Model file for the job. Use its own axes, mm. A direction names the side the tool comes from. Give positions to 0.01 mm unless a question says otherwise; leave off trailing zeros. Write each loop counter-clockwise with the first axis right and the second up, starting at its lowest first coordinate (ties: lowest second). Pieces come first, ordered by that corner, then holes.
```python
from build123d import *

# Parameters (mm, degrees)
SKETCH2_R           = 18.415
BOSS_EXTRUDE1_DEPTH = 70.104
SKETCH3_R           = 6.0325
BOSS_EXTRUDE2_DEPTH = 5.715
SKETCH5_R           = 3.01625
BOSS_EXTRUDE3_DEPTH = 14.986


with BuildPart() as part:
    # Sketch2 → Boss-Extrude1 (new body)
    with BuildSketch(Plane.XY):
        Circle(SKETCH2_R)
    extrude(amount=BOSS_EXTRUDE1_DEPTH)

    # Sketch3 → Boss-Extrude2 (add)
    with BuildSketch(Plane.XY.offset(70.104)):
        with Locations((0, -7.239)):
            Circle(SKETCH3_R)
    extrude(amount=BOSS_EXTRUDE2_DEPTH)

    # Sketch5 → Boss-Extrude3 (add)
    with BuildSketch(Plane.XY.offset(75.819)):
        with Locations((0, -7.239)):
            Circle(SKETCH5_R)
    extrude(amount=BOSS_EXTRUDE3_DEPTH)


solid = part.part
```
1. Slice it at A-A, the plane x = 0. Write the cut outline in (y, z) (1 decimal), and give its area (3 significant figures).
Calculated:
outline: (-18.4, 0) - (18.4, 0) - (18.4, 70.1) - (-1.2, 70.1) - (-1.2, 75.8) - (-4.2, 75.8) - (-4.2, 90.8) - (-10.3, 90.8) - (-10.3, 75.8) - (-13.3, 75.8) - (-13.3, 70.1) - (-18.4, 70.1) - close
area: 2,740 mm2
2. Probe probe 1 along Z at (x, y) = (12, 13.5); probe 2 along X at (y, z) = (-10.5, 53); probe 3 along X at (y, z) = (2, 14.5). List the from-to ranges inside material, lowest first.
Calculated:
probe 1: z = 0 to 70.1
probe 2: x = -15.13 to 15.13
probe 3: x = -18.31 to 18.31
3. Which spindle directions (+Z, -Z, +X, -X, +Y, -Y) get a long thin tool onto all of the face, cutting with end or side? Do faces 1 (the cylindrical face through (-14.61, -11.21, 34.56)), 2 (the flat face through (1, -4, 75.819)). Say none if no direction does.
Calculated:
face 1: +Z, -Z
face 2: +Z
4. Slice it at D-D, the plane y = -9. Write the cut outline in (x, z) (3 decimals).
Calculated:
outline: (-16.066, 0) - (16.066, 0) - (16.066, 70.104) - (5.77, 70.104) - (5.77, 75.819) - (2.449, 75.819) - (2.449, 90.805) - (-2.449, 90.805) - (-2.449, 75.819) - (-5.77, 75.819) - (-5.77, 70.104) - (-16.066, 70.104) - close
5. Pin check, flat tips, straight feed: P1, Ø10, axis at x = 8.5, y = -1, coming from the +Z side; P2, Ø3, axis at y = -7, z = 26.5, coming from the -X side; P3, Ø12, axis at y = 13, z = 33, coming from the +X side. Stop position of each tip, or through.
Calculated:
P1: stops at z = 75.82
P2: stops at x = -17.57
P3: stops at x = 17.03
6. Slice it at C-C, the plane z = 58.5. Write the cut outline in (x, y) (3 decimals), and give its area (3 significant figures).
Calculated:
outline: circle Ø36.83 at (0, 0)
area: 1,070 mm2
7. Slice it at B-B, the plane y = 0. Write the cut outline in (x, z) (3 decimals), and give its area (3 significant figures).
Calculated:
outline: (-18.415, 0) - (18.415, 0) - (18.415, 70.104) - (-18.415, 70.104) - close
area: 2,580 mm2
